```python
from build123d import *

# Parameters (mm, degrees)
F0_R     = 4.867648
F0_R_2   = 5.105565
F0_R_3   = 4.788046
F0_R_4   = 4.770591
F0_R_5   = 5.049327
F1_DEPTH = 6.35
F2_R     = 4.925574
F3_DEPTH = 25.4


with BuildPart() as f1:
    # F0 (on Top) → F1 (new body)
    with BuildSketch(Plane.XY):
        with BuildLine():
            Line((134.823743, 51.212785), (-68.884257, 51.212785))
            ThreePointArc((-68.884257, 51.212785), (-73.374385, 49.352913), (-75.234257, 44.862785))
            Line((-75.234257, 44.862785), (-75.234257, -54.451215))
            ThreePointArc((-75.234257, -54.451215), (-73.374385, -58.941343), (-68.884257, -60.801215))
            Line((-68.884257, -60.801215), (134.823743, -60.801215))
            ThreePointArc((134.823743, -60.801215), (139.313871, -58.941343), (141.173743, -54.451215))
            Line((141.173743, -54.451215), (141.173743, 44.862785))
            ThreePointArc((141.173743, 44.862785), (139.313871, 49.352913), (134.823743, 51.212785))
        make_face()
        with Locations((-63.880457, -47.656715)):
            Circle(F0_R, mode=Mode.SUBTRACT)
        with Locations((32.969743, -47.656715)):
            Circle(F0_R_2, mode=Mode.SUBTRACT)
        with Locations((129.819943, -47.656715)):
            Circle(F0_R_3, mode=Mode.SUBTRACT)
        with Locations((-63.880457, 38.068285)):
            Circle(F0_R_4, mode=Mode.SUBTRACT)
        with Locations((129.819943, 38.068285)):
            Circle(F0_R_5, mode=Mode.SUBTRACT)
    extrude(amount=F1_DEPTH)

    # F2 (on face) → F3 (cut)
    with BuildSketch(Plane.XY.offset(6.35)):
        with Locations((32.969743, 38.068285)):
            Circle(F2_R)
    extrude(amount=-F3_DEPTH, mode=Mode.SUBTRACT)


solid = f1.part
```
Here's how the part is built. I have some questions about the finished solid (model axes, mm). Give positions to 0.01 mm unless a question says otherwise; leave off trailing zeros. Loops run counter-clockwise (first coordinate to the right, second up) from the corner with the lowest first, then second, coordinate; pieces in that order, holes last. Notation, with made-up numbers: (56, 7) -> (79, 7) arc R23 ccw to (79, 35) -> close; hole circle Ø3 at (-9, 77). An arc over 180 degrees is marked (long way). Use one line per item in the form item = value. Start each with the question number.
1) Imagine slicing it at C-C (z = 4.75). Please give me the cut outline in (x, y).
2) Imagine slicing it at A-A (x = 128). Please give me the cut outline in (y, z).
3) Thinking about a two-plate mould opening in X: for faces 1 (the face through (139.264, -58.99, 3.131)), 2 (the face through (37.84, -46.12, 3.13)), 3 (the face through (31, -4, 6.35)), which applies, +X half, -X half, draft (parallel to the pull), parting line (faces both ways), or undercut?
4) Please list where these lines run through material, in increasing order: line 1 along X through (y, z) = (-51, 1.25); line 2 along Y through (x, z) = (35, 2.25).
5) Imagine slicing it at B-B (y = 40.5). Please give me the cut outline in (x, z).
6) For P1, Ø5.5, axis at x = -63.88, y = 38.07, coming from the +Z side, with a flat end and sliding along its axis, tell me the tip position at first contact or that it passes through.
Check values:
q1.outline = (-75.23, -54.45) arc R6.35 ccw to (-68.88, -60.8) -> (134.82, -60.8) arc R6.35 ccw to (141.17, -54.45) -> (141.17, 44.86) arc R6.35 ccw to (134.82, 51.21) -> (-68.88, 51.21) arc R6.35 ccw to (-75.23, 44.86) -> close; hole circle Ø9.74 at (-63.88, -47.66); hole circle Ø9.54 at (-63.88, 38.07); hole circle Ø10.21 at (32.97, -47.66); hole circle Ø9.85 at (32.97, 38.07); hole circle Ø10.1 at (129.82, 38.07); hole circle Ø9.58 at (129.82, -47.66)
q2.outline = (-60.8, 0) -> (-52.09, 0) -> (-52.09, 6.35) -> (-60.8, 6.35) -> close; (-43.23, 0) -> (33.36, 0) -> (33.36, 6.35) -> (-43.23, 6.35) -> close; (42.78, 0) -> (51.21, 0) -> (51.21, 6.35) -> (42.78, 6.35) -> close
q3.face_1 = +X half
q3.face_2 = undercut
q3.face_3 = draft
q4.line_1 = -75.23 to -67.42, -60.34 to 29.11, 36.83 to 126.39, 133.25 to 141.17
q4.line_2 = -60.8 to -52.34, -42.97 to 33.58, 42.56 to 51.21
q5.outline = (-75.23, 0) -> (-67.98, 0) -> (-67.98, 6.35) -> (-75.23, 6.35) -> close; (-59.78, 0) -> (28.69, 0) -> (28.69, 6.35) -> (-59.78, 6.35) -> close; (37.25, 0) -> (125.39, 0) -> (125.39, 6.35) -> (37.25, 6.35) -> close; (134.25, 0) -> (141.17, 0) -> (141.17, 6.35) -> (134.25, 6.35) -> close
q6.P1 = through
